Read the model definition and answer for the solid it produces. Units are mm, in the model's axes. Face numbers are marked on the shaded views. A direction names the side the tool comes from. Coordinates: 2 decimals unless noted, no trailing zeros. Order: outer loops, then holes, each group sorted by start corner. A loop starts at its lowest first (then second) coordinate and runs counter-clockwise, first axis right, second up.
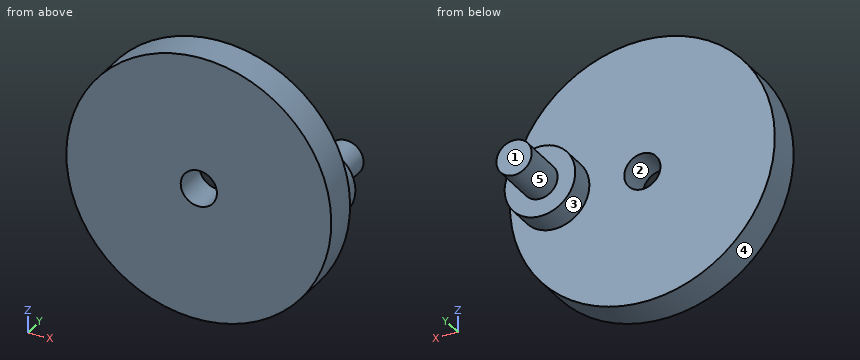
from build123d import *

# Parameters (mm, degrees)
SKETCH_1_R          = 30
EXTRUDE_1_DEPTH     = 8
SKETCH_2_R          = 4.1
CUT_EXTRUDE_1_DEPTH = 44.17406629
SKETCH_3_R          = 8
EXTRUDE_2_DEPTH     = 6
SKETCH_4_R          = 4
EXTRUDE_3_DEPTH     = 11


with BuildPart() as part:
    # 草图1 → 凸台-拉伸1 (new body)
    with BuildSketch(Plane(origin=(0, 0, 0), x_dir=(1, 0, 0), z_dir=(0, 1, 0))):
        with Locations(Location((0, 0, 0), (0, 0, 270))):
            Circle(SKETCH_1_R)
    extrude(amount=EXTRUDE_1_DEPTH)

    # 草图2 → 切除-拉伸1 (cut, through all)
    with BuildSketch(Plane(origin=(0, 8, 0), x_dir=(1, 0, 0), z_dir=(0, 1, 0))):
        with Locations(Location((0, 0, 0), (0, 0, 270))):
            Circle(SKETCH_2_R)
    extrude(amount=-CUT_EXTRUDE_1_DEPTH, mode=Mode.SUBTRACT)

    # 草图3 → 凸台-拉伸2 (add)
    with BuildSketch(Plane(origin=(0, 8, 0), x_dir=(1, 0, 0), z_dir=(0, 1, 0))):
        with Locations(Location((20, 0, 0), (0, 0, 270))):
            Circle(SKETCH_3_R)
    extrude(amount=EXTRUDE_2_DEPTH)

    # 草图4 → 凸台-拉伸3 (add)
    with BuildSketch(Plane(origin=(0, 14, 0), x_dir=(1, 0, 0), z_dir=(0, 1, 0))):
        with Locations(Location((20, 0, 0), (0, 0, 270))):
            Circle(SKETCH_4_R)
    extrude(amount=EXTRUDE_3_DEPTH)


solid = part.part
Q1. The part is cut by section A-A, the plane x = 0. Determine the outline of the cut face in (y, z).
Q2. Which of the six approach directions +Z, -Z, +X, -X, +Y, -Y give full straight-line access (tool end or side, diameter ignored) to the marked faces 4 and 5?
Q3. Determine the mould class of the marked faces 1, 2 and 3 for opening direction Z: +Z half, -Z half, draft (parallel to the pull), parting line (faces both ways), or undercut.
Q4. The part is cut by section C-C, the plane y = 3. Determine the outline of the cut face in (x, z), then the cut area to 3 significant figures.
Q5. The part is cut by section B-B, the plane z = 0. Determine the outline of the cut face in (x, y), then the cut area to 3 significant figures.
Q6. Each of these flat-tipped pins is pushed along its axis until it touches: P1, Ø10, axis at x = -11, y = 14, coming from the +Z side; P2, Ø8, axis at x = 10, y = 9, coming from the +Z side; P3, Ø8, axis at x = 3, y = 4.5, coming from the -Z side; P4, Ø12, axis at x = -15, z = 13.5, coming from the +Y side. Where does it stop, or does it pass through?
Q7. The part is cut by section D-D, the plane x = 20. Determine the outline of the cut face in (y, z).
Q8. Straight lines are drawn through the part: L1, parallel to X at y = 5.5, z = 0; L2, parallel to Y at x = 4, z = 27; L3, parallel to Y at x = 26.5, z = 0.5. For each, find the intervals that lie inside material, in ascending order.
Computed values:
1. outline: (0, -30) - (8, -30) - (8, -4.1) - (0, -4.1) - close; (0, 4.1) - (8, 4.1) - (8, 30) - (0, 30) - close
2. face 4: +Y, -Y
2. face 5: +Y
3. face 1: draft
3. face 2: undercut
3. face 3: parting line
4. outline: circle Ø60 at (0, 0); hole circle Ø8.2 at (0, 0)
4. area: 2,770 mm2
5. outline: (-30, 0) - (-4.1, 0) - (-4.1, 8) - (-30, 8) - close; (4.1, 0) - (30, 0) - (30, 8) - (28, 8) - (28, 14) - (24, 14) - (24, 25) - (16, 25) - (16, 14) - (12, 14) - (12, 8) - (4.1, 8) - close
5. area: 598 mm2
6. P1: passes through
6. P2: stops at z = 29.37
6. P3: stops at z = -30
6. P4: stops at y = 8
7. outline: (0, -22.36) - (8, -22.36) - (8, -8) - (14, -8) - (14, -4) - (25, -4) - (25, 4) - (14, 4) - (14, 8) - (8, 8) - (8, 22.36) - (0, 22.36) - close
8. L1: x = -30 to -4.1, 4.1 to 30
8. L2: y = 0 to 8
8. L3: y = 0 to 14
